Could you check a few things on this model? Use its own coordinates, in mm. Face numbers are marked on the shaded views. A direction names the side the tool comes from. Round coordinates to 2 decimals unless told otherwise and drop trailing zeros. Order: outer loops, then holes, each group sorted by start corner. A loop starts at its lowest first (then second) coordinate and runs counter-clockwise, first axis right, second up. Notation, with made-up numbers: (15, 67.25) -> (36, 67.25) arc R18 cw to (36, 99.25) -> close; hole circle Ø2 at (25.25, 7.25). An arc over 180 degrees is marked (long way). One line per question, with ' | ' between items.
```python
from build123d import *

# Parameters (mm, degrees)
SALIENTE_EXTRUIR1_DEPTH = 88.9
CROQUIS4_R              = 3.25
CORTAR_EXTRUIR1_DEPTH   = 112.44204772
REDONDEO6_R             = 3
REDONDEO7_R             = 3
ESCALA2_SCALE           = 1.05
SALIENTE_EXTRUIR2_DEPTH = 93.345
REDONDEO8_R             = 10
REDONDEO9_R             = 10
REDONDEO12_R            = 10
REDONDEO13_R            = 10
REDONDEO14_R            = 10
REDONDEO16_R            = 10
REDONDEO17_R            = 3
CROQUIS20_R             = 2.78
CORTAR_EXTRUIR7_DEPTH   = 10
ESCALA3_SCALE           = 0.9


with BuildPart() as part:
    # Croquis1 → Saliente-Extruir1 (new body)
    with BuildSketch(Plane(origin=(0, 0, 0), x_dir=(1, 0, 0), z_dir=(0, 1, 0))):
        Polygon((1.696358741, -16.064461222), (13.335, -27.703102481), (0, -50.8), (-13.335, -27.703102481), (-1.696358741, -16.064461222), (-14.760410887, 6.563140847), (-30.659090512, 2.303102481), (-43.994090512, 25.4), (-17.324090512, 25.4), (-13.064052146, 9.501320374), (13.064052146, 9.501320374), (17.324090512, 25.4), (43.994090512, 25.4), (30.659090512, 2.303102481), (14.760410887, 6.563140847), align=None)
    extrude(amount=SALIENTE_EXTRUIR1_DEPTH)

    # Croquis4 → Cortar-Extruir1 (cut, through all)
    with BuildSketch(Plane(origin=(0, 88.9, 0), x_dir=(1, 0, 0), z_dir=(0, 1, 0))):
        with Locations(Location((0, 0, 0), (0, 0, 270))):
            Circle(CROQUIS4_R)
    extrude(amount=-CORTAR_EXTRUIR1_DEPTH, mode=Mode.SUBTRACT)

    # Redondeo6
    redondeo6_edges = [part.edges().sort_by_distance(p)[0] for p in [
        (-1.696358741, 44.45, 16.064461222),
        (-14.760410887, 44.45, -6.563140847),
        (-13.064052146, 44.45, -9.501320374),
        (13.064052146, 44.45, -9.501320374),
        (1.696358741, 44.45, 16.064461222),
    ]]
    fillet(redondeo6_edges, radius=REDONDEO6_R)

    # Redondeo7
    redondeo7_edges = [part.edges().sort_by_distance(p)[0] for p in [
        (-13.335, 44.45, 27.703102481),
        (-30.659090512, 44.45, -2.303102481),
        (-17.324090512, 44.45, -25.4),
        (17.324090512, 44.45, -25.4),
        (30.659090512, 44.45, -2.303102481),
        (13.335, 44.45, 27.703102481),
    ]]
    fillet(redondeo7_edges, radius=REDONDEO7_R)


with BuildPart() as part_1:
    # Escala2: scaled about (-0.00814633, 44.45, 0.003262785)
    add(part.part.scale(ESCALA2_SCALE).moved(Location((0.000407317, -2.2225, -0.000163139))))

    # Croquis9 → Saliente-Extruir2 (add, through all)
    with BuildSketch(Plane(origin=(0, 91.1225, 0), x_dir=(1, 0, 0), z_dir=(0, 1, 0))):
        with BuildLine():
            Line((-37.193388788, 26.670163139), (-37.193388788, 61.670162712))
            ThreePointArc((-37.193388788, 61.670162712), (-35.728922694, 65.205696618), (-32.193388788, 66.670162712))
            Line((-32.193388788, 66.670162712), (-17.564301381, 66.670162712))
            Line((-17.564301381, 66.670162712), (-17.564301381, 61.670162712))
            Line((-17.564301381, 61.670162712), (-32.193388788, 61.670162712))
            Line((-32.193388788, 61.670162712), (-32.193388788, 26.670163139))
            Line((-32.193388788, 26.670163139), (-37.193388788, 26.670163139))
        make_face()
        with BuildLine():
            Line((-69.504104547, -2.954490104), (-39.193215784, 14.545509683))
            Line((-39.193215784, 14.545509683), (-41.693215784, 18.875636702))
            Line((-41.693215784, 18.875636702), (-72.004104547, 1.375636915))
            ThreePointArc((-72.004104547, 1.375636915), (-74.333733678, -1.660394878), (-73.834231566, -5.454490104))
            Line((-73.834231566, -5.454490104), (-66.519687862, -18.123651433))
            Line((-66.519687862, -18.123651433), (-62.189560843, -15.623651433))
            Line((-62.189560843, -15.623651433), (-69.504104547, -2.954490104))
        make_face()
        with BuildLine():
            Line((32.193388788, 61.670162712), (32.193388788, 26.670163139))
            Line((32.193388788, 26.670163139), (37.193388788, 26.670163139))
            Line((37.193388788, 26.670163139), (37.193388788, 61.670162712))
            ThreePointArc((37.193388788, 61.670162712), (35.728922694, 65.205696618), (32.193388788, 66.670162712))
            Line((32.193388788, 66.670162712), (17.564301381, 66.670162712))
            Line((17.564301381, 66.670162712), (17.564301381, 61.670162712))
            Line((17.564301381, 61.670162712), (32.193388788, 61.670162712))
        make_face()
        with BuildLine():
            Line((39.193733196, 14.545210955), (41.693733196, 18.875337974))
            Line((41.693733196, 18.875337974), (72.004621958, 1.375338188))
            ThreePointArc((72.004621958, 1.375338188), (74.33425109, -1.660693606), (73.834748977, -5.454788831))
            Line((73.834748977, -5.454788831), (66.520205273, -18.123950161))
            Line((66.520205273, -18.123950161), (62.190078254, -15.623950161))
            Line((62.190078254, -15.623950161), (69.504621958, -2.954788831))
            Line((69.504621958, -2.954788831), (39.193733196, 14.545210955))
        make_face()
        with BuildLine():
            Line((37.31123317, -58.715373881), (7.000344407, -41.215374094))
            Line((7.000344407, -41.215374094), (4.500344407, -45.545501113))
            Line((4.500344407, -45.545501113), (34.81123317, -63.0455009))
            ThreePointArc((34.81123317, -63.0455009), (38.605328395, -63.545003012), (41.641360189, -61.215373881))
            Line((41.641360189, -61.215373881), (48.955903893, -48.546212551))
            Line((48.955903893, -48.546212551), (44.625776874, -46.046212551))
            Line((44.625776874, -46.046212551), (37.31123317, -58.715373881))
        make_face()
        with BuildLine():
            Line((-6.999826996, -41.215075367), (-4.499826996, -45.545202386))
            Line((-4.499826996, -45.545202386), (-34.810715758, -63.045202172))
            ThreePointArc((-34.810715758, -63.045202172), (-38.604810984, -63.544704284), (-41.640842777, -61.215075153))
            Line((-41.640842777, -61.215075153), (-48.955386481, -48.545913824))
            Line((-48.955386481, -48.545913824), (-44.625259462, -46.045913824))
            Line((-44.625259462, -46.045913824), (-37.310715758, -58.715075153))
            Line((-37.310715758, -58.715075153), (-6.999826996, -41.215075367))
        make_face()
    extrude(amount=-SALIENTE_EXTRUIR2_DEPTH)

    # Redondeo8
    # the kernel refuses this fillet: 10 mm, written as the material it adds along each edge
    with BuildSketch(Plane(origin=(-37.193388788, 91.1225, -26.670163139), x_dir=(-1, 0, 0), z_dir=(0, -1, 0))) as redondeo8_piece_1_section:
        with BuildLine():
            CenterArc((10, 9.949874264), REDONDEO8_R, 180, 84.260823378)
            Line((0, 9.949874264), (-0.2, 9.949874264))
            Line((-0.2, 9.949874264), (-0.2, 0))
            Line((-0.2, 0), (0, -0.2))
            ThreePointArc((0, -0.2), (4.499999466, -0.2), (8.979998912, -0.198997485))
            Line((8.979998912, -0.198997485), (8.999998933, 0))
        make_face()
    redondeo8_piece_1 = extrude(amount=93.345, mode=Mode.PRIVATE)
    redondeo8_piece_1 = split(redondeo8_piece_1, bisect_by=Plane(origin=(-45.471806186, 44.45, -25.420347259), z_dir=(0.8660254037844427, 0, -0.49999999999999306)), keep=Keep.TOP, mode=Mode.PRIVATE)
    add(redondeo8_piece_1)

    # Redondeo9
    # the kernel refuses this fillet: 10 mm, written as the material it adds along each edge
    with BuildSketch(Plane(origin=(37.193388788, 91.1225, -26.670163139), x_dir=(0, 0, -1), z_dir=(0, -1, 0))) as redondeo9_piece_1_section:
        with BuildLine():
            CenterArc((9.949956104, 10), REDONDEO9_R, 185.734485624, 84.265514376)
            Line((0, 9.000813566), (-0.198999122, 8.980829837))
            ThreePointArc((-0.198999122, 8.980829837), (-0.2, 4.500406783), (-0.2, 0))
            Line((-0.2, 0), (0, -0.2))
            Line((0, -0.2), (9.949956104, -0.2))
            Line((9.949956104, -0.2), (9.949956104, 0))
        make_face()
    redondeo9_piece_1 = extrude(amount=93.345, mode=Mode.PRIVATE)
    redondeo9_piece_1 = split(redondeo9_piece_1, bisect_by=Plane(origin=(45.472441412, 44.45, -25.420036516), z_dir=(-0.8660254037844312, 0, -0.5000000000000131)), keep=Keep.TOP, mode=Mode.PRIVATE)
    add(redondeo9_piece_1)

    # Redondeo12
    # the kernel refuses this fillet: 10 mm, written as the material it adds along each edge
    with BuildSketch(Plane(origin=(4.500437971, 91.1225, 45.545555132), x_dir=(0.8660254037844384, 0, 0.5000000000000003), z_dir=(0, -1, 0))) as redondeo12_piece_1_section:
        with BuildLine():
            CenterArc((9.949880533, 10), REDONDEO12_R, 185.738817437, 84.261182563)
            Line((0, 9.000061308), (-0.198997611, 8.980062535))
            ThreePointArc((-0.198997611, 8.980062535), (-0.2, 4.500030654), (-0.2, 0))
            Line((-0.2, 0), (0, -0.2))
            Line((0, -0.2), (9.949880533, -0.2))
            Line((9.949880533, -0.2), (9.949880533, 0))
        make_face()
    redondeo12_piece_1 = extrude(amount=93.345, mode=Mode.PRIVATE)
    redondeo12_piece_1 = split(redondeo12_piece_1, bisect_by=Plane(origin=(-0.721187955, 44.45, 52.089997188), z_dir=(0.8660254037844385, 0, -0.5000000000000004)), keep=Keep.TOP, mode=Mode.PRIVATE)
    add(redondeo12_piece_1)

    # Redondeo13
    # the kernel refuses this fillet: 10 mm, written as the material it adds along each edge
    with BuildSketch(Plane(origin=(41.693826759, 91.1225, -18.875283955), x_dir=(0.500000000000013, 0, -0.8660254037844312), z_dir=(0, -1, 0))) as redondeo13_piece_1_section:
        with BuildLine():
            CenterArc((10, 9.94994984), REDONDEO13_R, 180, 84.265155193)
            Line((0, 9.94994984), (-0.2, 9.94994984))
            Line((-0.2, 9.94994984), (-0.2, 0))
            Line((-0.2, 0), (0, -0.2))
            ThreePointArc((0, -0.2), (4.500375595, -0.2), (8.980766214, -0.198998997))
            Line((8.980766214, -0.198998997), (9.00075119, 0))
        make_face()
    redondeo13_piece_1 = extrude(amount=93.345, mode=Mode.PRIVATE)
    redondeo13_piece_1 = redondeo13_piece_1 - Plane(origin=(47.193388788, 44.45, -36.620119243), x_dir=(0, 0, -1), z_dir=(0, 1, 0)) * Cylinder(10, 227, mode=Mode.PRIVATE)
    add(redondeo13_piece_1)

    # Redondeo14
    # the kernel refuses this fillet: 10 mm, written as the material it adds along each edge
    with BuildSketch(Plane(origin=(-4.499826996, 91.1225, 45.545202386), x_dir=(0.4999999999984365, 0, 0.8660254037853413), z_dir=(0, -1, 0))) as redondeo14_piece_1_section:
        with BuildLine():
            CenterArc((10, 9.949921458), REDONDEO14_R, 180, 84.263528066)
            Line((0, 9.949921459), (-0.2, 9.949921459))
            Line((-0.2, 9.949921459), (-0.2, 0))
            Line((-0.2, 0), (0, -0.2))
            ThreePointArc((0, -0.2), (4.500234312, -0.2), (8.980477997, -0.198998429))
            Line((8.980477997, -0.198998429), (9.000468625, 0))
        make_face()
    redondeo14_piece_1 = extrude(amount=93.345, mode=Mode.PRIVATE)
    redondeo14_piece_1 = redondeo14_piece_1 - Plane(origin=(8.117287277, 44.45, 59.180749436), x_dir=(0.866025403784329, 0, 0.50000000000019), z_dir=(0, 1, 0)) * Cylinder(10, 227, mode=Mode.PRIVATE)
    add(redondeo14_piece_1)

    # Redondeo16
    # the kernel refuses this fillet: 10 mm, written as the material it adds along each edge
    with BuildSketch(Plane(origin=(-41.693215784, 91.1225, -18.875636702), x_dir=(-0.8660254037844388, 0, 0.4999999999999999), z_dir=(0, -1, 0))) as redondeo16_piece_1_section:
        with BuildLine():
            CenterArc((9.949908926, 10), REDONDEO16_R, 185.737190303, 84.262809697)
            Line((0, 9.000343874), (-0.198998178, 8.980350751))
            ThreePointArc((-0.198998178, 8.980350751), (-0.2, 4.500171937), (-0.2, 0))
            Line((-0.2, 0), (0, -0.2))
            Line((0, -0.2), (9.949908926, -0.2))
            Line((9.949908926, -0.2), (9.949908926, 0))
        make_face()
    redondeo16_piece_1 = extrude(amount=93.345, mode=Mode.PRIVATE)
    redondeo16_piece_1 = redondeo16_piece_1 - Plane(origin=(-47.193388788, 44.45, -36.620037403), x_dir=(-1, 0, 0), z_dir=(0, 1, 0)) * Cylinder(10, 227, mode=Mode.PRIVATE)
    add(redondeo16_piece_1)

    # Redondeo17
    redondeo17_edges = [part_1.edges().sort_by_distance(p)[0] for p in [
        (15.498838747, 44.45, -6.891461029),
    ]]
    fillet(redondeo17_edges, radius=REDONDEO17_R)

    # Croquis20 → Cortar-Extruir7 (cut)
    with BuildSketch(Plane(origin=(-57.737537171, 0, 33.334782628), x_dir=(0.5000000000000017, 0, 0.8660254037844378), z_dir=(-0.8660254037844377, 0, 0.5000000000000016))):
        with Locations((25.193388788, 4.7775)):
            Circle(CROQUIS20_R)
        with Locations((25.193388788, 84.1225)):
            Circle(CROQUIS20_R)
        with Locations((-25.193388788, 84.1225)):
            Circle(CROQUIS20_R)
        with Locations((-25.193388788, 4.7775)):
            Circle(CROQUIS20_R)
    extrude(amount=-CORTAR_EXTRUIR7_DEPTH, mode=Mode.SUBTRACT)


with BuildPart() as part_2:
    # Escala3: scaled about (0.076174525, 44.45, -0.044030198)
    add(part_1.part.scale(ESCALA3_SCALE).moved(Location((0.007617452, 4.445, -0.00440302))))


solid = part_2.part
```
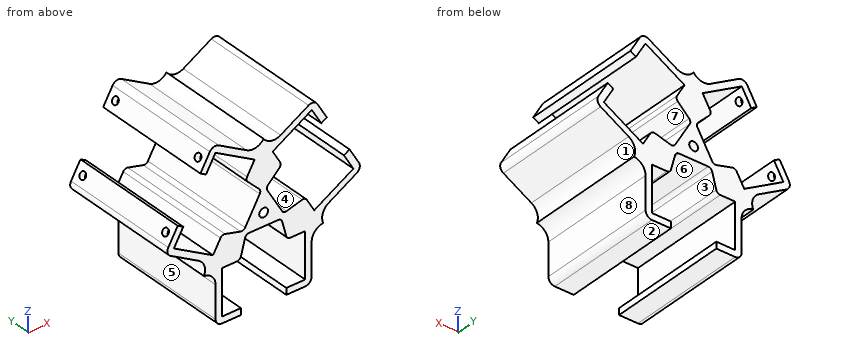
1. I'm going to push flat-ended pins straight in: pin 1 (18 mm diameter, centred on y = 43.5, z = -48.5, fed in from +X); pin 2 (1.5 mm diameter, centred on x = 7, y = 17.5, fed in from -Z); pin 3 (25 mm diameter, centred on y = 46.5, z = -39.5, fed in from +X). Where does each tip first touch, or does it pass through?
From the geometry:
pin 1: stops at x = 33.48 | pin 2: stops at z = -8.98 | pin 3: stops at x = 35.74
2. On a 3-axis mill with a long thin cutter (end or side, diameter ignored), from which of +Z, -Z, +X, -X, +Y, -Y can I reach the whole of each face in a straight line? I mean the marked faces 4, 5, 6, 7 and 8. Say none if no direction works.
From the geometry:
face 4: +Y, -Y | face 5: -Z, -X, +Y, -Y | face 6: -Z, +Y, -Y | face 7: +X, +Y, -Y | face 8: -Z, +X, +Y, -Y
3. I want a section at C-C on z = 39. List the corners of the cut face in (x, y) for me.
From the geometry:
outline: (-9.6, 2.44) -> (9.62, 2.44) -> (9.62, 86.46) -> (-9.6, 86.46) -> close
4. I need wall thicknesses on probe 1 along X at (y, z) = (23, -45); probe 2 along X at (y, z) = (33, 13.5); probe 3 along Z at (x, y) = (19.5, 7.5). Which ranges of each line are inside material? Lowest first, please.
From the geometry:
probe 1: x = -33.47 to -28.97, 28.98 to 33.48 | probe 2: x = -61.48 to -56.28, -2.57 to 2.59, 56.3 to 61.5 | probe 3: z = -60.01 to -55.51, -24.01 to -4.72, 44.71 to 49.9
5. I want a section at B-B on z = 1. List the corners of the cut face in (x, y) for me, and give its area (3 significant figures).
From the geometry:
outline: (-66.73, 2.44) -> (-59.68, 2.44) -> (-59.68, 86.46) -> (-66.73, 86.46) -> close; (-9.78, 2.44) -> (-2.89, 2.44) -> (-2.89, 86.46) -> (-9.78, 86.46) -> close; (2.91, 2.44) -> (9.8, 2.44) -> (9.8, 86.46) -> (2.91, 86.46) -> close; (59.7, 2.44) -> (66.75, 2.44) -> (66.75, 86.46) -> (59.7, 86.46) -> close | area: 2,340 mm²
6. I want a section at A-A on z = -35.5. List the corners of the cut face in (x, y) for me.
From the geometry:
outline: (-33.47, 2.44) -> (-28.97, 2.44) -> (-28.97, 86.46) -> (-33.47, 86.46) -> close; (28.98, 2.44) -> (33.48, 2.44) -> (33.48, 86.46) -> (28.98, 86.46) -> close
7. If we mould it in two halves opening along X, with no side actions, what happens to the marked faces 1, 2 and 3? For each: pulls with the +X half, pulls with the -X half, needs draft (parallel to the pull), parting line crosses it, or undercut.
From the geometry:
face 1: pulls with the +X half | face 2: needs draft | face 3: undercut
